```python
from build123d import *

# Parameters (mm, degrees)
SKETCH2_W          = 1.25
SKETCH2_H          = 11
SKETCH4_W          = 1.25
SKETCH4_H          = 11
SKETCH6_R          = 3.048
CUT_EXTRUDE1_DEPTH = 18.5000001


with BuildPart() as part:
    # Sketch1 → Revolve1 (revolve)
    with BuildSketch(Plane.XY):
        Polygon((0, 2.5), (0, 6), (6.3, 6), (6.3, 11), (7.9, 11), (7.9, 9.325), (15.9, 9.325), (15.9, 11), (17.5, 11), (17.5, 2.5), align=None)
    revolve(axis=Axis((0, 0, 0), (-1, 0, 0)))

    # Sketch2 → M3x0.5 Tapped Hole1 (revolve, cut)
    with BuildSketch(Plane(origin=(3.15, 0, 0), x_dir=(0, 0, -1), z_dir=(1, 0, 0))):
        with Locations((0.625, 5.5)):
            Rectangle(SKETCH2_W, SKETCH2_H)
    revolve(axis=Axis((3.15, -6.35, 0), (0, 1, 0)), mode=Mode.SUBTRACT)

    # Sketch4 → M3x0.5 Tapped Hole2 (revolve, cut)
    with BuildSketch(Plane.YZ.offset(3.15)):
        with Locations((0.625, 5.5)):
            Rectangle(SKETCH4_W, SKETCH4_H)
    revolve(axis=Axis((3.15, 0, -6.35), (0, 0, 1)), mode=Mode.SUBTRACT)

    # Sketch6 → Cut-Extrude1 (cut, through all)
    with BuildSketch(Plane(origin=(17.5, 0, 0), x_dir=(0, 0, -1), z_dir=(1, 0, 0))):
        Circle(SKETCH6_R)
    extrude(amount=-CUT_EXTRUDE1_DEPTH, mode=Mode.SUBTRACT)


solid = part.part
```
CAD build for the part. Positions are in the model's coordinates, mm. A direction names the side the tool comes from. Give positions to 0.01 mm unless a question says otherwise; leave off trailing zeros. Loops run counter-clockwise (first coordinate to the right, second up) from the corner with the lowest first, then second, coordinate; pieces in that order, holes last. Notation, with made-up numbers: (-32.75, 33) -> (-13.75, 33) arc R10 cw to (-13.75, 46) -> close; hole circle Ø8 at (59, 60.5). An arc over 180 degrees is marked (long way). Use a Markdown table: item, result.
1. Wall check: L1, parallel to Z at x = 11.5, y = 0 (3 decimals); L2, parallel to X at y = 3.6, z = 0. Give the ranges that are in metal, low to high. Write a range as [from, to].
Check result:
| item | result |
|---|---|
| L1 | z = [-9.325, -3.048], [3.048, 9.325] |
| L2 | x = [0, 1.9], [4.4, 17.5] |
2. Slice it at D-D (x = 12.25). List the corners of the cut face in (y, z) (3 decimals), plus the area to 3 significant figures.
Check result:
| item | result |
|---|---|
| outline | circle Ø18.65 at (0, 0); hole circle Ø6.096 at (0, 0) |
| area | 244 mm^2 |
3. Slice it at C-C (z = 5). List the corners of the cut face in (x, y).
Check result:
| item | result |
|---|---|
| outline | (0, -3.32) -> (6.3, -3.32) -> (6.3, -9.8) -> (7.9, -9.8) -> (7.9, -7.87) -> (15.9, -7.87) -> (15.9, -9.8) -> (17.5, -9.8) -> (17.5, 9.8) -> (15.9, 9.8) -> (15.9, 7.87) -> (7.9, 7.87) -> (7.9, 9.8) -> (6.3, 9.8) -> (6.3, 3.32) -> (0, 3.32) -> close; hole circle Ø2.5 at (3.15, 0) |
4. Slice it at B-B (x = 3.15). List the corners of the cut face in (y, z).
Check result:
| item | result |
|---|---|
| outline | (-1.25, 2.78) -> (-1.25, 5.87) arc R6 ccw (long way) to (5.87, -1.25) -> (2.78, -1.25) arc R3.05 cw (long way) to start; (1.25, 2.78) arc R3.05 cw to (2.78, 1.25) -> (5.87, 1.25) arc R6 ccw to (1.25, 5.87) -> close |
5. Slice it at A-A (z = 0). List the corners of the cut face in (x, y) (3 decimals).
Check result:
| item | result |
|---|---|
| outline | (0, -6) -> (6.3, -6) -> (6.3, -11) -> (7.9, -11) -> (7.9, -9.325) -> (15.9, -9.325) -> (15.9, -11) -> (17.5, -11) -> (17.5, -3.048) -> (0, -3.048) -> close; (0, 3.048) -> (1.9, 3.048) -> (1.9, 6) -> (0, 6) -> close; (4.4, 3.048) -> (17.5, 3.048) -> (17.5, 11) -> (15.9, 11) -> (15.9, 9.325) -> (7.9, 9.325) -> (7.9, 11) -> (6.3, 11) -> (6.3, 6) -> (4.4, 6) -> close |
6. Mould opens along Z. For faces 1 (the flat face through (6.3, -5, 5)), 2 (the cylindrical face through (8.9, -1.2, -2.8)), 3 (the cylindrical face through (1.91, 4.41, 0.16)), 4 (the cylindrical face through (3, -6, 0)) say: pulls with the +Z half, pulls with the -Z half, needs draft (parallel to the pull), parting line crosses it, or undercut.
Check result:
| item | result |
|---|---|
| face 1 | needs draft |
| face 2 | undercut |
| face 3 | undercut |
| face 4 | parting line crosses it |
7. Which spindle directions (+Z, -Z, +X, -X, +Y, -Y) get a long thin tool onto all of the face, cutting with end or side? Do faces 5 (the flat face through (7.9, -8.2, -4.9)), 6 (the cylindrical face through (16.71, -2.38, 10.74)), 7 (the cylindrical face through (1.91, -0.16, 4.41)). Say none if no direction does.
Check result:
| item | result |
|---|---|
| face 5 | none |
| face 6 | +X, -X |
| face 7 | +Z |
8. Flat gauge pins, fed straight in: pin 1 (1.5 mm diameter, centred on x = 6, y = -5.5, fed in from -Z); pin 2 (1.5 mm diameter, centred on x = 2, y = 0, fed in from +Z); pin 3 (3 mm diameter, centred on x = 13, y = -5, fed in from +Z); pin 4 (10 mm diameter, centred on x = 15, y = -0.5, fed in from -Z). Where does each tip first touch, or does it go through?
Check result:
| item | result |
|---|---|
| pin 1 | stops at z = -9.89 |
| pin 2 | stops at z = 6 |
| pin 3 | stops at z = 8.64 |
| pin 4 | stops at z = -11 |
